Read the model definition and answer for the solid it produces. Units are mm, in the model's axes. Face numbers are marked on the shaded views. Coordinates: 2 decimals unless noted, no trailing zeros. Write each loop counter-clockwise with the first axis right and the second up, starting at its lowest first coordinate (ties: lowest second). Pieces come first, ordered by that corner, then holes.
(1) Find the intervals of material crossed by probe 1 along Z at (x, y) = (-0.5, 18); probe 2 along Y at (x, z) = (0, 4.55); probe 3 along Y at (x, z) = (0, 9), in increasing order.
(2) Section A-A on z = 4.75 is taken. Write down the section's boundary in (x, y).
(3) Section B-B on x = 4.5 is taken. Write down the section's boundary in (y, z), then the cut area to 3 significant figures.
(4) The mould has two halves that part along X. Classify the marked faces 1, 2 and 3: +X half, -X half, draft (parallel to the pull), parting line (faces both ways), or undercut.
(5) Given pin 1 (1.5 mm diameter, centred on y = 148, z = -2, fed in from +X); pin 2 (2 mm diameter, centred on x = -5, z = 3, fed in from -Y); pin 3 (1 mm diameter, centred on y = 39.5, z = 7.5, fed in from -X), each flat-ended and moving along its own axis, determine where each tip first touches the part or whether it passes through.
(6) Section C-C on y = 60 is taken. Write down the section's boundary in (x, z), then the cut area to 3 significant figures.
from build123d import *

# Parameters (mm, degrees)
SKETCH1_R               = 11
BOSS_EXTRUDE1_DEPTH     = 216.66667
BOSS_EXTRUDE2_START     = 216.66667
SKETCH2_R               = 6.8
BOSS_EXTRUDE2_DEPTH     = 19.8
CUT_EXTRUDE1_START      = -1.44
SKETCH3_R               = 0.5
CUT_EXTRUDE1_DEPTH      = 9
CUT_EXTRUDE2_START      = -1.4
SKETCH4_R               = 0.5
CUT_EXTRUDE2_DEPTH      = 9
SKETCH6_R               = 7
CUT_EXTRUDE3_DEPTH      = 20
CUT_EXTRUDE4_DEPTH      = 237.977817671
CUT_EXTRUDE4_DEPTH_BACK = 237.977817671
SKETCH7_R               = 0.5
CUT_EXTRUDE5_DEPTH      = 237.97781768
CUT_EXTRUDE5_DEPTH_BACK = 237.97781768
SKETCH10_R              = 0.5


with BuildPart() as part:
    # Sketch1 → Boss-Extrude1 (new body)
    with BuildSketch(Plane(origin=(0, 0, 0), x_dir=(1, 0, 0), z_dir=(0, 1, 0))):
        with Locations(Location((0, 0, 0), (0, 0, 270))):
            Circle(SKETCH1_R)
    extrude(amount=BOSS_EXTRUDE1_DEPTH)

    # Sketch2 → Boss-Extrude2 (add)
    with BuildSketch(Plane(origin=(0, 0, 0), x_dir=(1, 0, 0), z_dir=(0, 1, 0)).offset(BOSS_EXTRUDE2_START)):
        with Locations(Location((0, 0, 0), (0, 0, 90))):
            Circle(SKETCH2_R)
    extrude(amount=BOSS_EXTRUDE2_DEPTH)

    # Sketch3 → Cut-Extrude1 (cut)
    with BuildSketch(Plane.XY.offset(CUT_EXTRUDE1_START)):
        with Locations((0, 231.66667)):
            Circle(SKETCH3_R)
    cut_extrude1 = extrude(amount=-CUT_EXTRUDE1_DEPTH, mode=Mode.SUBTRACT)

    # Mirror1: Cut-Extrude1 across plane
    add(cut_extrude1.mirror(Plane.XY), mode=Mode.SUBTRACT)

    # Sketch4 → Cut-Extrude2 (cut)
    with BuildSketch(Plane(origin=(0, 0, 0), x_dir=(0, 0, -1), z_dir=(1, 0, 0)).offset(CUT_EXTRUDE2_START)):
        with Locations((0, 226.66667)):
            Circle(SKETCH4_R)
    cut_extrude2 = extrude(amount=-CUT_EXTRUDE2_DEPTH, mode=Mode.SUBTRACT)

    # Mirror2: Cut-Extrude2 across plane
    add(cut_extrude2.mirror(Plane(origin=(0, 0, 0), x_dir=(0, 0, 1), z_dir=(1, 0, 0))), mode=Mode.SUBTRACT)

    # Sketch6 → Cut-Extrude3 (cut)
    with BuildSketch(Plane(origin=(0, 0, 0), x_dir=(1, 0, 0), z_dir=(0, 1, 0))):
        with Locations(Location((0, 0, 0), (0, 0, 270))):
            Circle(SKETCH6_R)
    extrude(amount=CUT_EXTRUDE3_DEPTH, mode=Mode.SUBTRACT)

    # Sketch7 → Cut-Extrude4 (cut, two sides: drawn at the far end of the back side and taken through both)
    with BuildSketch(Plane(origin=(0, 0, 0), x_dir=(0, 0, -1), z_dir=(1, 0, 0)).offset(-CUT_EXTRUDE4_DEPTH_BACK)):
        with Locations((0, 10)):
            Circle(SKETCH7_R)
    extrude(amount=CUT_EXTRUDE4_DEPTH + CUT_EXTRUDE4_DEPTH_BACK, mode=Mode.SUBTRACT)

    # Sketch10 → Cut-Extrude5 (cut, two sides: drawn at the far end of the back side and taken through both)
    with BuildSketch(Plane.XY.offset(-CUT_EXTRUDE5_DEPTH_BACK)):
        with Locations((0, 5)):
            Circle(SKETCH10_R)
    extrude(amount=CUT_EXTRUDE5_DEPTH + CUT_EXTRUDE5_DEPTH_BACK, mode=Mode.SUBTRACT)


solid = part.part
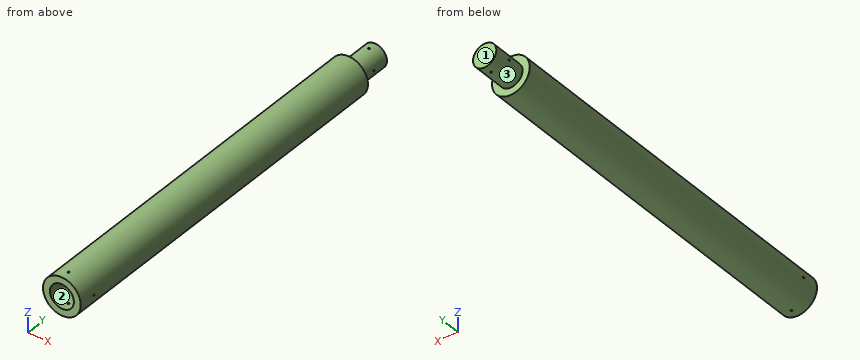
Response:
1. probe 1: z = -10.99 to -6.98, 6.98 to 10.99
1. probe 2: y = 20 to 231.17, 232.17 to 236.47
1. probe 3: y = 0 to 4.5, 5.5 to 216.67
2. outline: (-9.92, 0) - (-5.14, 0) - (-5.14, 20) - (5.14, 20) - (5.14, 0) - (9.92, 0) - (9.92, 216.67) - (4.87, 216.67) - (4.87, 236.47) - (-4.87, 236.47) - (-4.87, 216.67) - (-9.92, 216.67) - close; hole circle Ø1 at (0, 231.67)
3. outline: (0, -10.04) - (216.67, -10.04) - (216.67, -5.1) - (236.47, -5.1) - (236.47, 5.1) - (216.67, 5.1) - (216.67, 10.04) - (0, 10.04) - (0, 5.36) - (20, 5.36) - (20, -5.36) - (0, -5.36) - close; hole circle Ø1 at (226.67, 0)
3. area: 4,340 mm2
4. face 1: draft
4. face 2: undercut
4. face 3: parting line
5. pin 1: stops at x = 10.93
5. pin 2: stops at y = 20
5. pin 3: stops at x = -8.49
6. outline: circle Ø22 at (0, 0)
6. area: 380 mm2
